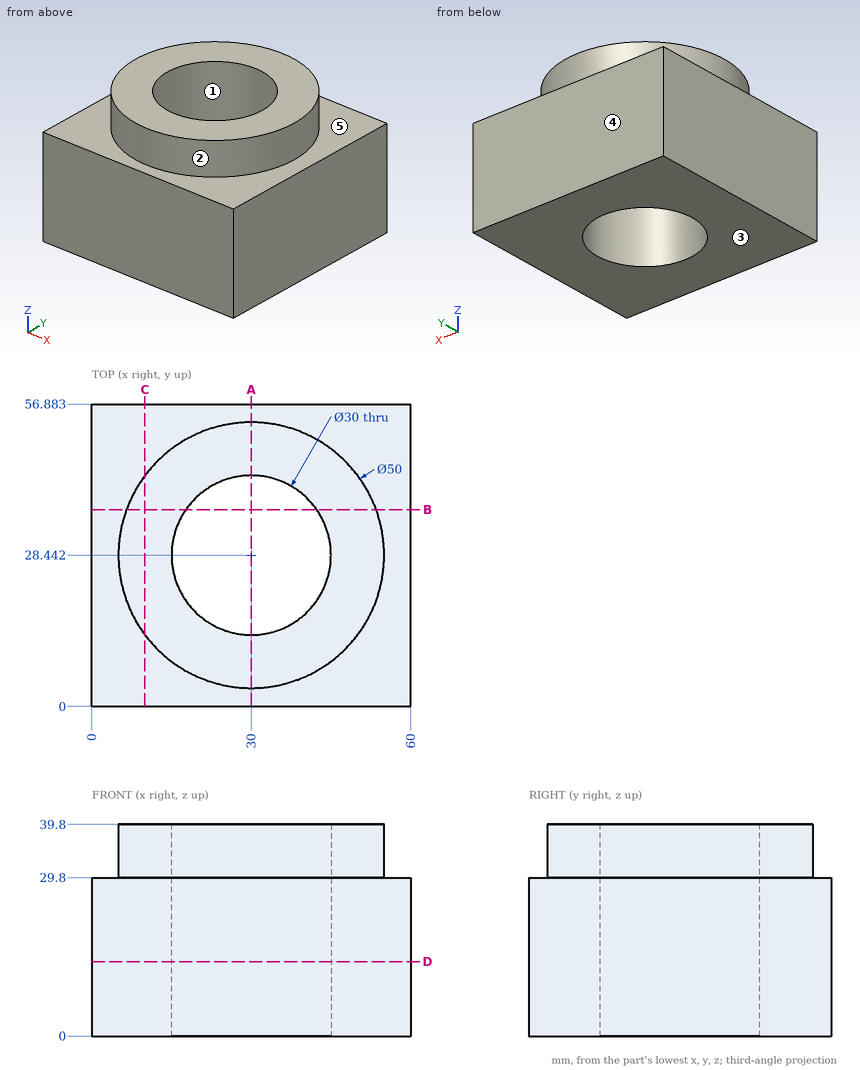
Part print with two shaded views. Sizes in mm from the minimum x, y, z corner. A direction names the side the tool comes from. Round coordinates to 2 decimals unless told otherwise and drop trailing zeros. Order: outer loops, then holes, each group sorted by start corner. A loop starts at its lowest first (then second) coordinate and runs counter-clockwise, first axis right, second up. Notation, with made-up numbers: M 11.25,52 L 30.25,52 A18 ccw 30.25,83 Z; hole C -34.5,46.25 d4. An arc over 180 degrees is marked long. Answer in a Markdown table with one row per item. Add a question column.
Q1. 3-axis set-ups, long thin cutter, end or side, ignore diameter. For the marked faces 4 and 5: which of +Z, -Z, +X, -X, +Y, -Y reach the whole face in a straight line?
Q2. Mould opens along X. For the marked faces 1, 2 and 3 say: +X half, -X half, draft (parallel to the pull), parting line (faces both ways), or undercut.
Q3. Pin check, flat tips, straight feed: pin 1 (2 mm diameter, centred on y = 38.5, z = 35, fed in from +X); pin 2 (1.5 mm diameter, centred on x = 29.5, z = 35, fed in from -Y); pin 3 (5 mm diameter, centred on x = 19.5, y = 34.5, fed in from +Z); pin 4 (5 mm diameter, centred on x = 17.5, z = 31, fed in from +Y). Stop position of each tip, or through.
Q4. Cut at A-A on x = 30. Give the cut face in (y, z).
Q5. Cut at C-C on x = 10. Give the cut face in (y, z), and give its area (4 significant figures).
Q6. Cut at B-B on y = 37. Give the cut face in (x, z).
Q7. Cut at D-D on z = 14. Give the cut face in (x, y).
Q8. Wall check: L1, parallel to Y at x = 30, z = 27; L2, parallel to Y at x = 30, z = 31.5; L3, parallel to X at y = 23.5, z = 17. Give the ranges that are in metal, low to high. Write a range as from..to.
Established:
| question | item | result |
|---|---|---|
| 1 | face 4 | +Z, -Z, +X, -X, +Y |
| 1 | face 5 | +Z |
| 2 | face 1 | undercut |
| 2 | face 2 | parting line |
| 2 | face 3 | draft |
| 3 | pin 1 | stops at x = 53.3 |
| 3 | pin 2 | stops at y = 3.44 |
| 3 | pin 3 | passes through |
| 3 | pin 4 | stops at y = 56.88 |
| 4 | outline | M 0,0 L 13.44,0 L 13.44,39.8 L 3.44,39.8 L 3.44,29.8 L 0,29.8 Z; M 43.44,0 L 56.88,0 L 56.88,29.8 L 53.44,29.8 L 53.44,39.8 L 43.44,39.8 Z |
| 5 | outline | M 0,0 L 56.88,0 L 56.88,29.8 L 43.44,29.8 L 43.44,39.8 L 13.44,39.8 L 13.44,29.8 L 0,29.8 Z |
| 5 | area | 1,995 mm2 |
| 6 | outline | M 0,0 L 17.68,0 L 17.68,39.8 L 6.51,39.8 L 6.51,29.8 L 0,29.8 Z; M 42.32,0 L 60,0 L 60,29.8 L 53.49,29.8 L 53.49,39.8 L 42.32,39.8 Z |
| 7 | outline | M 0,0 L 60,0 L 60,56.88 L 0,56.88 Z; hole C 30,28.44 d30 |
| 8 | L1 | y = 0..13.44, 43.44..56.88 |
| 8 | L2 | y = 3.44..13.44, 43.44..53.44 |
| 8 | L3 | x = 0..15.84, 44.16..60 |
